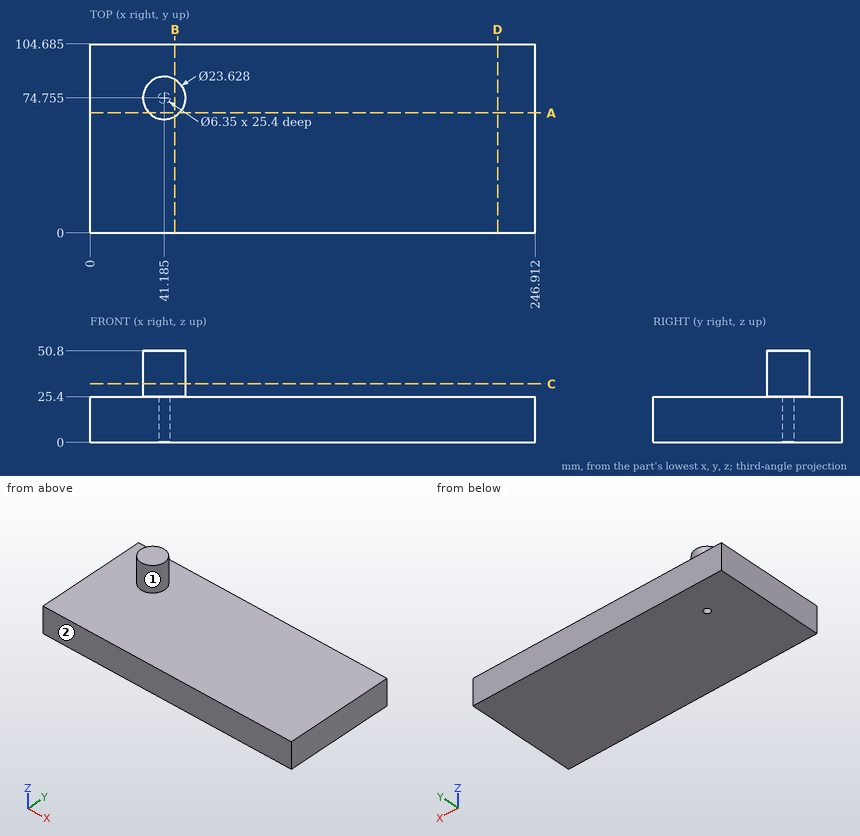
Print and shaded views of the part. All mm, measured from the part's lowest x, y and z. A direction names the side the tool comes from. Give positions to 0.01 mm unless a question says otherwise; leave off trailing zeros. Write each loop counter-clockwise with the first axis right and the second up, starting at its lowest first coordinate (ties: lowest second). Pieces come first, ordered by that corner, then holes. Notation, with made-up numbers: M -25,82 L -9,82 A34 cw -9,118 Z; hole C 50,23 d5. An arc over 180 degrees is marked long. Use a Markdown table: item, result.
1) Cut at D-D (x = 226). List the corners of the cut face in (y, z) (1 decimal), and give its area (3 significant figures).
Responses:
| item | result |
|---|---|
| outline | M 0,0 L 104.7,0 L 104.7,25.4 L 0,25.4 Z |
| area | 2,660 mm2 |
2) Drill centre lines: line 1 (Z direction, x = 189, y = 40.5); line 2 (X direction, y = 74.5, z = 26); line 3 (X direction, y = 68.5, z = 35). Where is each one in solid material? Low to high. Write a range as from..to.
Responses:
| item | result |
|---|---|
| line 1 | z = 0..25.4 |
| line 2 | x = 29.37..53 |
| line 3 | x = 31.16..51.21 |
3) Tool access for the marked faces 1 and 2: list every direction of +Z, -Z, +X, -X, +Y, -Y with a clear straight run to the whole face (end or side of a thin tool).
Responses:
| item | result |
|---|---|
| face 1 | +Z |
| face 2 | +Z, -Z, +X, -X, -Y |
4) Pin check, flat tips, straight feed: pin 1 (4 mm diameter, centred on x = 140.5, y = 71.5, fed in from +Z); pin 2 (4 mm diameter, centred on x = 41.18, y = 74.76, fed in from -Z); pin 3 (4 mm diameter, centred on y = 59, z = 37, fed in from +X). Stop position of each tip, or through.
Responses:
| item | result |
|---|---|
| pin 1 | stops at z = 25.4 |
| pin 2 | stops at z = 25.4 |
| pin 3 | passes through |
5) Cut at A-A (y = 66.5). List the corners of the cut face in (x, z).
Responses:
| item | result |
|---|---|
| outline | M 0,0 L 246.91,0 L 246.91,25.4 L 49.64,25.4 L 49.64,50.8 L 32.73,50.8 L 32.73,25.4 L 0,25.4 Z |
6) Cut at C-C (z = 32.5). List the corners of the cut face in (x, y) (1 decimal).
Responses:
| item | result |
|---|---|
| outline | C 41.2,74.8 d23.6 |
7) Cut at B-B (x = 47). List the corners of the cut face in (y, z) (1 decimal).
Responses:
| item | result |
|---|---|
| outline | M 0,0 L 104.7,0 L 104.7,25.4 L 85,25.4 L 85,50.8 L 64.5,50.8 L 64.5,25.4 L 0,25.4 Z |
